Part model, mm, in its own coordinate system. Face numbers are marked on the shaded views. A direction names the side the tool comes from. Round coordinates to 2 decimals unless told otherwise and drop trailing zeros. Write each loop counter-clockwise with the first axis right and the second up, starting at its lowest first coordinate (ties: lowest second). Pieces come first, ordered by that corner, then holes.
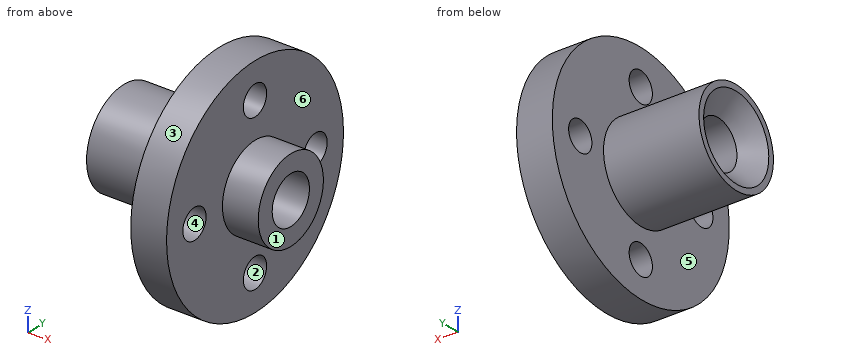
from build123d import *

# Parameters (mm, degrees)
SKETCH1_R           = 9.5
SKETCH1_R_2         = 1.25
SKETCH1_R_3         = 4
SKETCH1_R_4         = 3.5
BOSS_EXTRUDE1_DEPTH = 3
SKETCH1_3_R         = 3.5
SKETCH1_3_R_2       = 2
BOSS_EXTRUDE2_DEPTH = 6
BOSS_EXTRUDE3_START = -8
SKETCH1_4_R         = 4
SKETCH1_4_R_2       = 3.5
SKETCH1_4_R_3       = 2
BOSS_EXTRUDE3_DEPTH = 8


with BuildPart() as part:
    # Sketch1 → Boss-Extrude1 (new body)
    # profile 1 of 2: a face of its own
    with BuildSketch(Plane(origin=(0, 0, 0), x_dir=(0, 0, -1), z_dir=(1, 0, 0))):
        Circle(SKETCH1_R)
        with Locations((-6.5, 0)):
            Circle(SKETCH1_R_2, mode=Mode.SUBTRACT)
        with Locations((0, -6.5)):
            Circle(SKETCH1_R_2, mode=Mode.SUBTRACT)
        with Locations((6.5, 0)):
            Circle(SKETCH1_R_2, mode=Mode.SUBTRACT)
        with Locations((0, 6.5)):
            Circle(SKETCH1_R_2, mode=Mode.SUBTRACT)
        Circle(SKETCH1_R_3, mode=Mode.SUBTRACT)
    # profile 2 of 2: a face of its own
    with BuildSketch(Plane(origin=(0, 0, 0), x_dir=(0, 0, -1), z_dir=(1, 0, 0))):
        Circle(SKETCH1_R_3)
        Circle(SKETCH1_R_4, mode=Mode.SUBTRACT)
    extrude(amount=BOSS_EXTRUDE1_DEPTH)

    # Sketch1<3> → Boss-Extrude2 (add)
    with BuildSketch(Plane(origin=(0, 0, 0), x_dir=(0, 0, -1), z_dir=(1, 0, 0))):
        Circle(SKETCH1_3_R)
        Circle(SKETCH1_3_R_2, mode=Mode.SUBTRACT)
    extrude(amount=BOSS_EXTRUDE2_DEPTH)

    # Sketch1<4> → Boss-Extrude3 (add)
    # profile 1 of 2: a face of its own
    with BuildSketch(Plane(origin=(0, 0, 0), x_dir=(0, 0, -1), z_dir=(1, 0, 0)).offset(BOSS_EXTRUDE3_START)):
        Circle(SKETCH1_4_R)
        Circle(SKETCH1_4_R_2, mode=Mode.SUBTRACT)
    # profile 2 of 2: a face of its own
    with BuildSketch(Plane(origin=(0, 0, 0), x_dir=(0, 0, -1), z_dir=(1, 0, 0)).offset(BOSS_EXTRUDE3_START)):
        Circle(SKETCH1_4_R_2)
        Circle(SKETCH1_4_R_3, mode=Mode.SUBTRACT)
    extrude(amount=BOSS_EXTRUDE3_DEPTH)

    # Cut-Extrude1 cone 1 section (through the dimple's axis) → Cut-Extrude1 (revolve, cut)
    with BuildSketch(Plane(origin=(-8, 0, 0), x_dir=(0, 0, 1), z_dir=(0, 1, 0))):
        Polygon((0, 0), (3.5, 0), (0, 3.5), align=None)
    revolve(axis=Axis((-8, 0, 0), (1, 0, 0)), mode=Mode.SUBTRACT)


solid = part.part
Q1. Two-plate mould, pull along Y, no slides. Class the marked faces 1, 2 and 3: released by +Y, released by -Y, zero draft, split by the parting line, or undercut.
Q2. Saw through at C-C, the plane y = 7.5. Write the cut outline in (x, z).
Q3. Wall check: line 1 (Y direction, x = 1.1, z = 0); line 2 (X direction, y = -6.5, z = 5.5); line 3 (Z direction, x = -7, y = -0.5). Give the ranges that are in metal, low to high.
Q4. Tool access for the marked faces 4, 5 and 6: list every direction of +Z, -Z, +X, -X, +Y, -Y with a clear straight run to the whole face (end or side of a thin tool).
Q5. Saw through at A-A, the plane y = 0. Write the cut outline in (x, z), and give its area (4 significant figures).
Q6. Saw through at D-D, the plane z = 5.5. Write the cut outline in (x, y), and give its area (3 significant figures).
Q7. Drop flat-ended pins along their axis: P1, Ø4.5, axis at y = 0, z = 0, coming from the -X side; P2, Ø3, axis at y = 6.5, z = 0, coming from the -X side; P3, Ø2, axis at y = -3.5, z = -4, coming from the +X side; P4, Ø9.5, axis at y = 2.5, z = 3.5, coming from the +X side. Give the stop position or say it passes through.
Computed:
1. face 1: zero draft
1. face 2: undercut
1. face 3: split by the parting line
2. outline: (0, -5.83) - (3, -5.83) - (3, -0.75) - (0, -0.75) - close; (0, 0.75) - (3, 0.75) - (3, 5.83) - (0, 5.83) - close
3. line 1: y = -9.5 to -7.75, -5.25 to -2, 2 to 5.25, 7.75 to 9.5
3. line 2: x = 0 to 3
3. line 3: z = -3.97 to -2.45, 2.45 to 3.97
4. face 4: +X, -X
4. face 5: -X
4. face 6: +X
5. outline: (-8, -4) - (0, -4) - (0, -5.25) - (3, -5.25) - (3, -3.5) - (6, -3.5) - (6, -2) - (-6.5, -2) - (-8, -3.5) - close; (-8, 3.5) - (-6.5, 2) - (6, 2) - (6, 3.5) - (3, 3.5) - (3, 5.25) - (0, 5.25) - (0, 4) - (-8, 4) - close; (0, -9.5) - (3, -9.5) - (3, -7.75) - (0, -7.75) - close; (0, 7.75) - (3, 7.75) - (3, 9.5) - (0, 9.5) - close
5. area: 68.75 mm2
6. outline: (0, -7.75) - (3, -7.75) - (3, -0.75) - (0, -0.75) - close; (0, 0.75) - (3, 0.75) - (3, 7.75) - (0, 7.75) - close
6. area: 42.0 mm2
7. P1: stops at x = -6.75
7. P2: stops at x = 0
7. P3: stops at x = 3
7. P4: stops at x = 6
